Can you work these out from the model? Positions are in its coordinate system, mm. A direction names the side the tool comes from. Coordinates: 2 decimals unless noted, no trailing zeros. Order: outer loops, then holes, each group sorted by start corner. A loop starts at its lowest first (then second) coordinate and runs counter-clockwise, first axis right, second up. Notation, with made-up numbers: (56.5, -31) -> (76.5, -31) arc R18 cw to (76.5, -17) -> close; hole circle Ø7 at (0.5, 63). An arc over 180 degrees is marked (long way). Answer as a JSON object with one key per item and string values. Group by question number.
(1) For pin 1 (2 mm diameter, centred on y = -11.5, z = 0.5, fed in from -X); pin 2 (5 mm diameter, centred on y = -4, z = 3.5, fed in from -X); pin 3 (4 mm diameter, centred on x = -3.5, z = -3, fed in from +Y), each with a flat end and sliding along its axis, tell me the tip position at first contact or that it passes through.
(2) I want a section at C-C, the plane y = 7.25. List the corners of the cut face in (x, z) for me (3 decimals).
(3) I want a section at B-B, the plane y = -1.5. List the corners of the cut face in (x, z) for me (3 decimals).
(4) I want a section at A-A, the plane y = -10. List the corners of the cut face in (x, z) for me (3 decimals), plus the area to 3 significant figures.
(5) If we mould it in two halves opening along X, with no side actions, what happens to faces 4 (the flat face through (3, 0, -1)), 5 (the cylindrical face through (-2.893, -6.281, -2.653)), 6 (the flat face through (0, -9.45, 0))? For each: pulls with the +X half, pulls with the -X half, needs draft (parallel to the pull), parting line crosses it, or undercut.
(6) I need wall thicknesses on line 1 (Y direction, x = -3.5, z = -2); line 2 (Z direction, x = 0, y = 3.5); line 3 (Y direction, x = -2.25, z = -2.25). Which ranges of each line are inside material? Lowest first, please.
(7) Which directions (+Z, -Z, +X, -X, +Y, -Y) give clear straight access to the entire face, cutting with the end or side of a thin tool? Please do faces 1 (the cylindrical face through (-0.45, 7.528, -2.026)), 2 (the cylindrical face through (-3.789, -1.578, 2.906)), 3 (the flat face through (-1, -3.2, -4)).
Autodesk Inventor part; units mm, degrees
ref_plane "YZ Plane" through (0, 0, 0) normal (1, 0, 0) x (0, 1, 0)
ref_plane "XZ Plane" through (0, 0, 0) normal (0, 1, 0) x (-1, 0, 0)
ref_plane "XY Plane" through (0, 0, 0) normal (0, 0, 1) x (1, 0, 0)
sketch "Boceto1" plane through (0, 0, 0) normal (0, 1, 0) x (-1, 0, 0)
  circle A0 centre (0, 0) radius 3
  dimension "d0" = 6
extrude "Extrusión1" add sketch "Boceto1" along normal blind 6
sketch "Boceto2" plane through (0, 6, 0) normal (0, 1, 0) x (1, 0, 0)
  circle A0 centre (0, 0) radius 2.075
  dimension "d3" = 4.15
extrude "Extrusión2" add sketch "Boceto2" along normal blind 3.6
chamfer "Chaflán1" distance 2 distance2 0.5 1 edges at (-2.075, 9.6, 0) measured on face at (0.6845, 9.6, -0.4587)
sketch "Boceto3" plane through (0, 0, 0) normal (0, -1, 0) x (1, 0, 0)
  circle A0 centre (0, 0) radius 0.075
  circle A1 centre (0, 0) radius 4.775
  dimension "d9" = 9.55
extrude "Extrusión3" add sketch "Boceto3" along normal blind 3.2
sketch "Boceto4" plane through (0, -3.2, 0) normal (0, -1, 0) x (1, 0, 0)
  circle A0 centre (0, 0) radius 3.925
  dimension "d12" = 7.85
extrude "Extrusión4" add sketch "Boceto4" along normal blind 6.25
thread "Rosca1"
chamfer "Chaflán2" distance 0.5 angle 45 1 edges at (3, 6, 0)
sketch "Boceto5" plane through (0, -9.45, 0) normal (0, -1, 0) x (1, 0, 0)
  circle A0 centre (0, 0) radius 0.075
  line L0 (0, 0) -> (2.5, 0)
  line L1 (0, 0) -> (-2.5, 0)
  line L2 (2.45, 1.275) -> (2.55, 1.275)
  line L3 (2.55, 1.275) -> (2.55, -1.275)
  line L4 (2.55, -1.275) -> (2.45, -1.275)
  line L5 (2.45, -1.275) -> (2.45, 1.275)
  line L6 (2.45, 1.275) -> (2.55, -1.275) construction
  line L7 (2.55, 1.275) -> (2.45, -1.275) construction
  line L8 (-2.55, 1.275) -> (-2.45, 1.275)
  line L9 (-2.45, 1.275) -> (-2.45, -1.275)
  line L10 (-2.45, -1.275) -> (-2.55, -1.275)
  line L11 (-2.55, -1.275) -> (-2.55, 1.275)
  line L12 (-2.55, 1.275) -> (-2.45, -1.275) construction
  line L13 (-2.45, 1.275) -> (-2.55, -1.275) construction
  dimension "d20" = 2.5
  dimension "d21" = 2.5
  dimension "d22" = 0.1
  dimension "d23" = 2.55
  dimension "d24" = 0.1
extrude "Extrusión5" add sketch "Boceto5" along normal blind 5.5 contours L9 L10 L11 L8 | L5 L2 L3 L4
properties part number "Interruptor_BlueRobotics"
Computed values:
{
 "1": {"pin 1": "stops at x = -2.55", "pin 2": "stops at x = -4.64", "pin 3": "stops at y = 5.89"},
 "2": {"outline": "circle Ø4.15 at (0, 0)"},
 "3": {"outline": "circle Ø9.55 at (0, 0); hole circle Ø0.15 at (0, 0)"},
 "4": {"outline": "(-2.55, -1.275) -> (-2.45, -1.275) -> (-2.45, 1.275) -> (-2.55, 1.275) -> close; (2.45, -1.275) -> (2.55, -1.275) -> (2.55, 1.275) -> (2.45, 1.275) -> close", "area": "0.510 mm2"},
 "5": {"face 4": "needs draft", "face 5": "parting line crosses it", "face 6": "undercut"},
 "6": {"line 1": "y = -3.2 to 0", "line 2": "z = -3 to 3", "line 3": "y = -9.45 to 0"},
 "7": {"face 1": "+Y", "face 2": "+Y, -Y", "face 3": "-Y"}
}
